Design review of the part built by this model. Coordinates are the model's own, in mm. A direction names the side the tool comes from. Give positions to 0.01 mm unless a question says otherwise; leave off trailing zeros. Order: outer loops, then holes, each group sorted by start corner. A loop starts at its lowest first (then second) coordinate and runs counter-clockwise, first axis right, second up. Notation, with made-up numbers: (83.5, -29) -> (132.5, -29) arc R21 ccw to (132.5, 3) -> close; hole circle Ø9 at (55.25, 88). An arc over 180 degrees is marked (long way). One line per item, written item: value. Start each with the question number.
1) Tool access review of faces 1 (the face through (-4.8, 22.6, 4.75)), 2 (the face through (4.123, 22.283, 2.849)): name each direction out of +Z, -Z, +X, -X, +Y, -Y from which nothing blocks a thin tool from reaching the whole face with its end or side.
2) Consider section C-C (y = 23.5). State the section outline as (x, z) points.
3) For pin 1 (2 mm diameter, centred on x = 5, y = -1, fed in from +Z); pin 2 (3.5 mm diameter, centred on x = 5.71, y = 23.5, fed in from -Z), all flat-tipped, find the tip position at first contact; note any pin that passes through.
4) The part is to be moulded in two halves that separate along X. For faces 3 (the face through (-4.787, 21.726, 2.849)), 4 (the face through (18.2, 6.4, 4)), 5 (the face through (6, 24, 1)), 6 (the face through (-19, 0, 2)), say which applies: released by +X, released by -X, zero draft, split by the parting line, or undercut.
5) Consider section B-B (x = 11.5). State the section outline as (y, z) points, plus the area to 3 significant figures.
6) Consider section D-D (y = -4). State the section outline as (x, z) points, plus the area to 3 significant figures.
7) Wall thickness on line 1 along Y through (x, z) = (-5.71, 3.3); line 2 along X through (y, z) = (-23.5, 1.85); line 3 along Y through (x, z) = (-9, 2.55): over which ranges is each line inside the solid? List them lowest first. Write a range as from..to.
8) Consider section A-A (z = 3.1). State how many separate pieces and enclosed holes the cut face has, plus the area to 3 significant figures.
from build123d import *

# Parameters (mm, degrees)
SKETCH034_W     = 38
SKETCH034_H     = 56
PAD020_DEPTH    = 4
SKETCH035_W     = 36
SKETCH035_H     = 54
POCKET008_DEPTH = 3
SKETCH036_W     = 10
SKETCH036_H     = 3
POCKET009_DEPTH = 5
SKETCH037_R     = 2
SKETCH037_R_2   = 1.1
PAD021_DEPTH    = 3.75
SKETCH039_W     = 5
SKETCH039_H     = 5.5
POCKET011_DEPTH = 5


with BuildPart() as part:
    # Sketch034 → Pad020 (new body)
    with BuildSketch(Plane.XY):
        Rectangle(SKETCH034_W, SKETCH034_H)
    extrude(amount=PAD020_DEPTH)

    # Sketch035 (on Face6 of Pad020) → Pocket008 (cut)
    with BuildSketch(Plane.XY.offset(4)):
        Rectangle(SKETCH035_W, SKETCH035_H)
    extrude(amount=-POCKET008_DEPTH, mode=Mode.SUBTRACT)

    # Sketch036 (on Face1 of Pocket008) → Pocket009 (cut)
    with BuildSketch(Plane(origin=(0, 28, 0), x_dir=(-1, 0, 0), z_dir=(0, 1, 0))):
        with Locations((0, 2.5)):
            Rectangle(SKETCH036_W, SKETCH036_H)
    extrude(amount=-POCKET009_DEPTH, mode=Mode.SUBTRACT)

    # Sketch037 (on Face14 of Pocket009) → Pad021 (join)
    with BuildSketch(Plane.XY.offset(1)):
        with Locations((-5.71, 23.5)):
            Circle(SKETCH037_R)
        with Locations((-5.71, 23.5)):
            Circle(SKETCH037_R_2, mode=Mode.SUBTRACT)
        with Locations((5.71, 23.5)):
            Circle(SKETCH037_R)
        with Locations((5.71, 23.5)):
            Circle(SKETCH037_R_2, mode=Mode.SUBTRACT)
    pad021 = extrude(amount=PAD021_DEPTH)

    # Mirrored010: Pad021 across XZ
    add(pad021.mirror(Plane.XZ))

    # Sketch039 (on Face6 of Mirrored010) → Pocket011 (cut)
    with BuildSketch(Plane.XY.offset(1)):
        with Locations((3.21, 13.75)):
            Rectangle(SKETCH039_W, SKETCH039_H)
    extrude(amount=-POCKET011_DEPTH, mode=Mode.SUBTRACT)


solid = part.part
Checked values:
1. face 1: +Z, +X, -X, +Y, -Y
1. face 2: +Z
2. outline: (-19, 0) -> (19, 0) -> (19, 4) -> (18, 4) -> (18, 1) -> (7.71, 1) -> (7.71, 4.75) -> (6.81, 4.75) -> (6.81, 1) -> (4.61, 1) -> (4.61, 4.75) -> (3.71, 4.75) -> (3.71, 1) -> (-3.71, 1) -> (-3.71, 4.75) -> (-4.61, 4.75) -> (-4.61, 1) -> (-6.81, 1) -> (-6.81, 4.75) -> (-7.71, 4.75) -> (-7.71, 1) -> (-18, 1) -> (-18, 4) -> (-19, 4) -> close
3. pin 1: stops at z = 1
3. pin 2: stops at z = 0
4. face 3: undercut
4. face 4: zero draft
4. face 5: undercut
4. face 6: released by -X
5. outline: (-28, 0) -> (28, 0) -> (28, 4) -> (27, 4) -> (27, 1) -> (-27, 1) -> (-27, 4) -> (-28, 4) -> close
5. area: 62.0 mm^2
6. outline: (-19, 0) -> (19, 0) -> (19, 4) -> (18, 4) -> (18, 1) -> (-18, 1) -> (-18, 4) -> (-19, 4) -> close
6. area: 44.0 mm^2
7. line 1: y = -28..-27, -25.5..-24.6, -22.4..-21.5, 21.5..22.4, 24.6..25.5, 27..28
7. line 2: x = -19..-18, -7.71..-6.81, -4.61..-3.71, 3.71..4.61, 6.81..7.71, 18..19
7. line 3: y = -28..-27, 27..28
8. separate pieces: 5
8. enclosed holes: 4
8. area: 209 mm^2
